from build123d import *

# Parameters (mm, degrees)
SKETCH1_R           = 2.1
SKETCH1_R_2         = 4
SKETCH1_R_3         = 8
BOSS_EXTRUDE1_DEPTH = 5


with BuildPart() as part:
    # Sketch1 → Boss-Extrude1 (new body)
    with BuildSketch(Plane.XY):
        Polygon((116.611470678, 15.338509317), (51.611470678, 15.338509317), (51.611470678, -6.661490683), (51.611470678, -24.661490683), (116.611470678, -24.661490683), (134.111470678, -24.661490683), (134.111470678, -6.661490683), align=None)
        with Locations((56.611470678, 10.338509317)):
            Circle(SKETCH1_R, mode=Mode.SUBTRACT)
        with Locations((111.611470678, 10.338509317)):
            Circle(SKETCH1_R, mode=Mode.SUBTRACT)
        with Locations((56.611470678, 0.338509317)):
            Circle(SKETCH1_R, mode=Mode.SUBTRACT)
        with Locations((111.611470678, 0.338509317)):
            Circle(SKETCH1_R, mode=Mode.SUBTRACT)
        with Locations((115.611470678, -12.661490683)):
            Circle(SKETCH1_R_2, mode=Mode.SUBTRACT)
        with Locations((90.611470678, -12.661490683)):
            Circle(SKETCH1_R_3, mode=Mode.SUBTRACT)
        with Locations((78.111470678, -12.661490683)):
            Circle(SKETCH1_R, mode=Mode.SUBTRACT)
        with Locations((103.111470678, -12.661490683)):
            Circle(SKETCH1_R, mode=Mode.SUBTRACT)
        with Locations((128.111470678, -12.661490683)):
            Circle(SKETCH1_R, mode=Mode.SUBTRACT)
    extrude(amount=BOSS_EXTRUDE1_DEPTH)


solid = part.part
Verification items for the finished model (mm, model axes). Give positions to 0.01 mm unless a question says otherwise; leave off trailing zeros. Write each loop counter-clockwise with the first axis right and the second up, starting at its lowest first coordinate (ties: lowest second). Pieces come first, ordered by that corner, then holes.
(1) Cross-section at D-D (z = 2). State how many separate pieces and enclosed holes the cut face has, plus the area to 3 significant figures.
(2) Mould release check, pull along Y, two halves, no side actions. Record for faces 1 (the face through (134.111, -16, 2)), 2 (the face through (125.484, 4.185, 2.465)), 3 (the face through (54.514, 0.431, 2.465)): +Y half, -Y half, draft (parallel to the pull), parting line (faces both ways), or undercut.
(3) Cross-section at A-A (y = -1). Enter the section's corners in (x, z).
(4) Cross-section at C-C (y = -5.5). Enter the section's corners in (x, z), plus the area to 3 significant figures.
(5) Material ranges on line 1 (Y direction, x = 90.5, z = 3.35); line 2 (Y direction, x = 56.5, z = 0.9); line 3 (X direction, y = -15, z = 3), recorded low to high.
(6) Cross-section at B-B (x = 94.5). Enter the section's corners in (y, z), plus the area to 3 significant figures.
Worked out:
1. separate pieces: 1
1. enclosed holes: 9
1. area: 2,760 mm2
2. face 1: draft
2. face 2: +Y half
2. face 3: undercut
3. outline: (51.61, 0) - (54.99, 0) - (54.99, 5) - (51.61, 5) - close; (58.23, 0) - (109.99, 0) - (109.99, 5) - (58.23, 5) - close; (113.23, 0) - (129.61, 0) - (129.61, 5) - (113.23, 5) - close
4. outline: (51.61, 0) - (87.05, 0) - (87.05, 5) - (51.61, 5) - close; (94.18, 0) - (133.19, 0) - (133.19, 5) - (94.18, 5) - close
4. area: 372 mm2
5. line 1: y = -24.66 to -20.66, -4.66 to 15.34
5. line 2: y = -24.66 to -1.76, 2.44 to 8.24, 12.44 to 15.34
5. line 3: x = 51.61 to 82.96, 98.26 to 112.37, 118.86 to 134.11
6. outline: (-24.66, 0) - (-19.65, 0) - (-19.65, 5) - (-24.66, 5) - close; (-5.67, 0) - (15.34, 0) - (15.34, 5) - (-5.67, 5) - close
6. area: 130 mm2
